Input: dimensioned drawing with shaded views. Units: mm. Origin: part minimum x, y, z. Give positions to 0.01 mm unless a question says otherwise; leave off trailing zeros. Write each loop counter-clockwise with the first axis right and the second up, starting at its lowest first coordinate (ties: lowest second). Pieces come first, ordered by that corner, then holes. Notation, with made-up numbers: M 55,15 L 101,15 A16 ccw 101,27 Z; hole C 88.25,-33 d4. An arc over 180 degrees is marked long. Use CSV: the item, a comma, the result in double quotes. Start each with the question number.
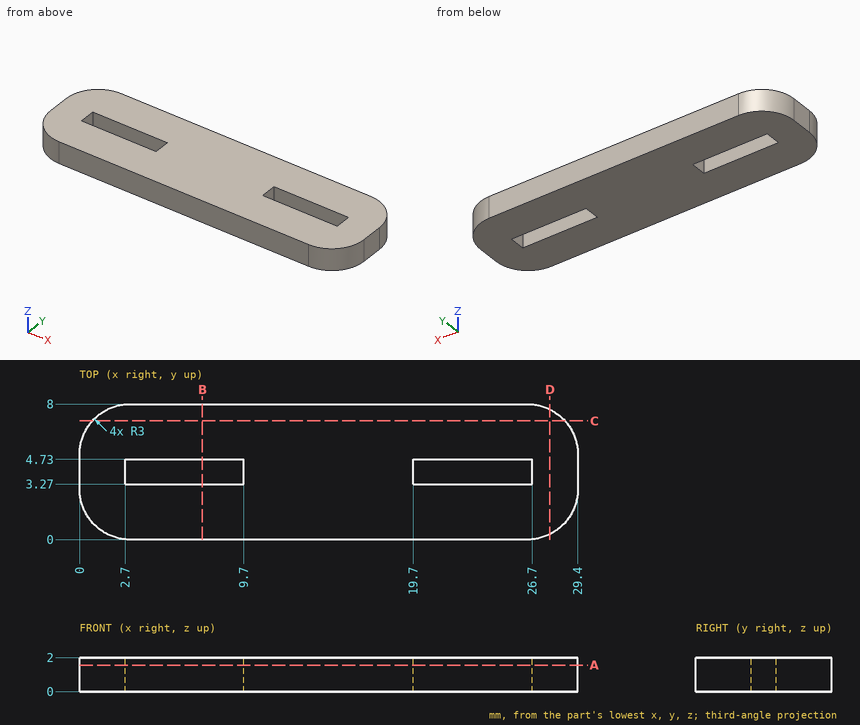
Item 1: Material intervals for probe 1 along Y at (x, z) = (26, 0.55); probe 2 along X at (y, z) = (4.25, 1.4); probe 3 along X at (y, z) = (2.5, 0.15), sorted ascending.
Item 2: Section C-C (y = 7). Return the cut outline in (x, z).
Item 3: Section A-A (z = 1.55). Return the cut outline in (x, y).
Item 4: Section B-B (x = 7.25). Return the cut outline in (y, z).
Item 5: Section D-D (x = 27.75). Return the cut outline in (y, z), plus the area to 3 significant figures.
Output values:
1,probe 1,"y = 0 to 3.27, 4.73 to 8"
1,probe 2,"x = 0 to 2.7, 9.7 to 19.7, 26.7 to 29.4"
1,probe 3,"x = 0.04 to 29.36"
2,outline,"M 0.76,0 L 28.64,0 L 28.64,2 L 0.76,2 Z"
3,outline,"M 0,3 A3 ccw 3,0 L 26.4,0 A3 ccw 29.4,3 L 29.4,5 A3 ccw 26.4,8 L 3,8 A3 ccw 0,5 Z; hole M 2.7,3.27 L 9.7,3.27 L 9.7,4.73 L 2.7,4.73 Z; hole M 19.7,3.27 L 26.7,3.27 L 26.7,4.73 L 19.7,4.73 Z"
4,outline,"M 0,0 L 3.27,0 L 3.27,2 L 0,2 Z; M 4.73,0 L 8,0 L 8,2 L 4.73,2 Z"
5,outline,"M 0.32,0 L 7.68,0 L 7.68,2 L 0.32,2 Z"
5,area,"14.7 mm2"
